Read the model definition and answer for the solid it produces. Units are mm, in the model's axes. Coordinates: 2 decimals unless noted, no trailing zeros. Loops run counter-clockwise (first coordinate to the right, second up) from the corner with the lowest first, then second, coordinate; pieces in that order, holes last.
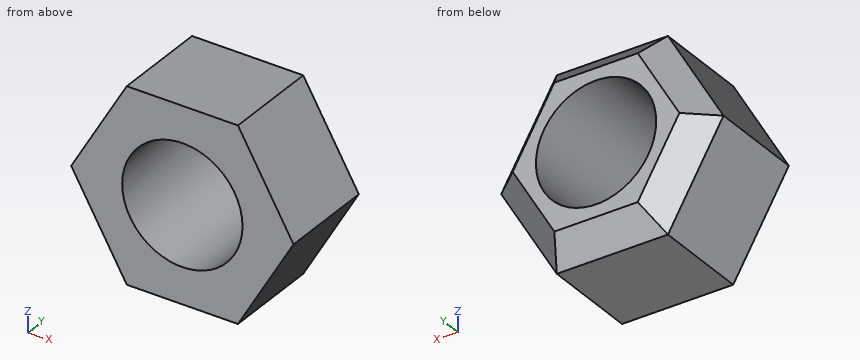
Autodesk Inventor part; units mm, degrees
ref_plane "YZ Plane" through (0, 0, 0) normal (1, 0, 0) x (0, 1, 0)
ref_plane "XZ Plane" through (0, 0, 0) normal (0, 1, 0) x (-1, 0, 0)
ref_plane "XY Plane" through (0, 0, 0) normal (0, 0, 1) x (1, 0, 0)
sketch "Szkic1" plane through (0, 0, 0) normal (0, 1, 0) x (-1, 0, 0)
  line L0 (-2.3094, -4) -> (-4.6188, 0)
  line L1 (-4.6188, 0) -> (-2.3094, 4)
  line L2 (-2.3094, 4) -> (2.3094, 4)
  line L3 (2.3094, 4) -> (4.6188, 0)
  line L4 (4.6188, 0) -> (2.3094, -4)
  line L5 (2.3094, -4) -> (-2.3094, -4)
  circle A0 centre (0, 0) radius 2.5
  dimension "d0" = 8
  dimension "d1" = 5
extrude "Wyciągnięcie proste1" add sketch "Szkic1" along normal blind 5
thread "Gwint1"
chamfer "Faza1" distance 1 angle 45 6 edges at (-3.4641, 5, 2) (0, 5, 4) (3.4641, 5, 2) (3.4641, 5, -2) (0, 5, -4) (-3.4641, 5, -2)
properties part number "M5_nut_5mm" material "Aluminium 6061"
Item 1: A cutting plane is placed at A-A on x = -1.5. Determine the outline of the cut face in (y, z), then the cut area to 3 significant figures.
Numbers:
outline: (0, -4) - (4, -4) - (5, -3) - (5, -2) - (0, -2) - close; (0, 2) - (5, 2) - (5, 3) - (4, 4) - (0, 4) - close
area: 19.0 mm2
Item 2: Given pin 1 (1.5 mm diameter, centred on y = 3, z = 3, fed in from +X); pin 2 (3 mm diameter, centred on y = 2, z = 2, fed in from -X); pin 3 (1.5 mm diameter, centred on y = 4.5, z = 1.5, fed in from +X), each flat-ended and moving along its own axis, determine where each tip first touches the part or whether it passes through.
Numbers:
pin 1: stops at x = 3.32
pin 2: stops at x = -4.33
pin 3: stops at x = 4.08
Item 3: A cutting plane is placed at C-C on z = -2. Determine the outline of the cut face in (x, y), then the cut area to 3 significant figures.
Numbers:
outline: (-3.46, 0) - (-1.5, 0) - (-1.5, 5) - (-2.31, 5) - (-3.46, 4) - close; (1.5, 0) - (3.46, 0) - (3.46, 4) - (2.31, 5) - (1.5, 5) - close
area: 18.5 mm2
Item 4: Find the intervals of material crossed by line 1 along Z through (x, y) = (0, 2.2); line 2 along Z through (x, y) = (-1, 3.95); line 3 along X through (y, z) = (3.75, -2), in increasing order.
Numbers:
line 1: z = -4 to -2.5, 2.5 to 4
line 2: z = -4 to -2.29, 2.29 to 4
line 3: x = -3.46 to -1.5, 1.5 to 3.46
Item 5: A cutting plane is placed at D-D on x = 2. Determine the outline of the cut face in (y, z), then the cut area to 3 significant figures.
Numbers:
outline: (0, -4) - (4, -4) - (4.54, -3.46) - (5, -2.54) - (5, -1.5) - (0, -1.5) - close; (0, 1.5) - (5, 1.5) - (5, 2.54) - (4.54, 3.46) - (4, 4) - (0, 4) - close
area: 23.8 mm2
Item 6: A cutting plane is placed at B-B on y = 0.9. Determine the outline of the cut face in (x, z), then the cut area to 3 significant figures.
Numbers:
outline: (-4.62, 0) - (-2.31, -4) - (2.31, -4) - (4.62, 0) - (2.31, 4) - (-2.31, 4) - close; hole circle Ø5 at (0, 0)
area: 35.8 mm2
